Work out the finished part from the listing and answer in its coordinate system (mm). A direction names the side the tool comes from. Coordinates: 2 decimals unless noted, no trailing zeros. Order: outer loops, then holes, each group sorted by start corner. A loop starts at its lowest first (then second) coordinate and runs counter-clockwise, first axis right, second up.
```python
from build123d import *

# Parameters (mm, degrees)
SKETCH1_R           = 1.65
SKETCH1_R_2         = 1.1
SKETCH1_R_3         = 1.4
SKETCH1_R_4         = 11
SKETCH1_W           = 28
SKETCH1_H           = 83
SKETCH1_W_2         = 6.35
SKETCH1_H_2         = 20
SKETCH1_W_3         = 20
SKETCH1_H_3         = 6.35
BOSS_EXTRUDE1_DEPTH = 6.35


with BuildPart() as part:
    # Sketch1 → Boss-Extrude1 (new body)
    with BuildSketch(Plane(origin=(0, 0, 0), x_dir=(1, 0, 0), z_dir=(0, 1, 0))):
        with BuildLine():
            Line((-110, 85), (-2.828427125, 192.171572875))
            ThreePointArc((-2.828427125, 192.171572875), (0, 193.343145751), (2.828427125, 192.171572875))
            Line((2.828427125, 192.171572875), (110, 85))
            Line((110, 85), (110, -85))
            Line((110, -85), (-110, -85))
            Line((-110, -85), (-110, 85))
        make_face()
        with Locations(Location((-39, 10.85, 0), (0, 0, 270))):
            Circle(SKETCH1_R, mode=Mode.SUBTRACT)
        with Locations(Location((-39, -10.85, 0), (0, 0, 90))):
            Circle(SKETCH1_R, mode=Mode.SUBTRACT)
        with Locations(Location((-89.294117647, -69, 0), (0, 0, 270))):
            Circle(SKETCH1_R, mode=Mode.SUBTRACT)
        with Locations(Location((89.294117647, -69, 0), (0, 0, 90))):
            Circle(SKETCH1_R, mode=Mode.SUBTRACT)
        with Locations(Location((-89.294117647, 69, 0), (0, 0, 90))):
            Circle(SKETCH1_R, mode=Mode.SUBTRACT)
        with Locations(Location((89.294117647, 69, 0), (0, 0, 270))):
            Circle(SKETCH1_R, mode=Mode.SUBTRACT)
        with Locations(Location((39, -10.85, 0), (0, 0, 270))):
            Circle(SKETCH1_R, mode=Mode.SUBTRACT)
        with Locations(Location((39, 10.85, 0), (0, 0, 90))):
            Circle(SKETCH1_R, mode=Mode.SUBTRACT)
        with Locations(Location((0, 157, 0), (0, 0, 270))):
            Circle(SKETCH1_R_2, mode=Mode.SUBTRACT)
        with Locations(Location((0, 141.75, 0), (0, 0, 270))):
            Circle(SKETCH1_R_2, mode=Mode.SUBTRACT)
        with Locations(Location((-3, -21, 0), (0, 0, 270))):
            Circle(SKETCH1_R_3, mode=Mode.SUBTRACT)
        with Locations(Location((-3, -70, 0), (0, 0, 270))):
            Circle(SKETCH1_R_3, mode=Mode.SUBTRACT)
        with Locations(Location((58.5, -70, 0), (0, 0, 270))):
            Circle(SKETCH1_R_3, mode=Mode.SUBTRACT)
        with Locations(Location((58.5, -21, 0), (0, 0, 270))):
            Circle(SKETCH1_R_3, mode=Mode.SUBTRACT)
        with Locations(Location((-6.75, 78.125, 0), (0, 0, 270))):
            Circle(SKETCH1_R, mode=Mode.SUBTRACT)
        with Locations(Location((6.75, 78.125, 0), (0, 0, 270))):
            Circle(SKETCH1_R, mode=Mode.SUBTRACT)
        with Locations(Location((6.75, 64.625, 0), (0, 0, 270))):
            Circle(SKETCH1_R, mode=Mode.SUBTRACT)
        with Locations(Location((-6.75, 64.625, 0), (0, 0, 270))):
            Circle(SKETCH1_R, mode=Mode.SUBTRACT)
        with Locations(Location((0, 173, 0), (0, 0, 270))):
            Circle(SKETCH1_R_4, mode=Mode.SUBTRACT)
        with Locations((-83, 0)):
            Rectangle(SKETCH1_W, SKETCH1_H, mode=Mode.SUBTRACT)
        with Locations((-104, 50)):
            Rectangle(SKETCH1_W_2, SKETCH1_H_2, mode=Mode.SUBTRACT)
        with Locations((-104, 0)):
            Rectangle(SKETCH1_W_2, SKETCH1_H_2, mode=Mode.SUBTRACT)
        with Locations((-104, -50)):
            Rectangle(SKETCH1_W_2, SKETCH1_H_2, mode=Mode.SUBTRACT)
        with Locations((50, -77.667136592)):
            Rectangle(SKETCH1_W_3, SKETCH1_H_3, mode=Mode.SUBTRACT)
        with Locations((0, -77.667136592)):
            Rectangle(SKETCH1_W_3, SKETCH1_H_3, mode=Mode.SUBTRACT)
        with Locations((-50, -77.667136592)):
            Rectangle(SKETCH1_W_3, SKETCH1_H_3, mode=Mode.SUBTRACT)
        with Locations((104, -50)):
            Rectangle(SKETCH1_W_2, SKETCH1_H_2, mode=Mode.SUBTRACT)
        with Locations((104, 50)):
            Rectangle(SKETCH1_W_2, SKETCH1_H_2, mode=Mode.SUBTRACT)
        with Locations((104, 0)):
            Rectangle(SKETCH1_W_2, SKETCH1_H_2, mode=Mode.SUBTRACT)
        with Locations((-50, 77.667136592)):
            Rectangle(SKETCH1_W_3, SKETCH1_H_3, mode=Mode.SUBTRACT)
        with Locations((50, 77.667136592)):
            Rectangle(SKETCH1_W_3, SKETCH1_H_3, mode=Mode.SUBTRACT)
        with Locations((83, 0)):
            Rectangle(SKETCH1_W, SKETCH1_H, mode=Mode.SUBTRACT)
    extrude(amount=BOSS_EXTRUDE1_DEPTH)


solid = part.part
```
1. Consider probe 1 along X at (y, z) = (4.75, 21); probe 2 along X at (y, z) = (5.75, -38); probe 3 along X at (y, z) = (6, 58) (3 decimals). Determine where each line is inside the solid, lowest interval first.
2. The mould has two halves that part along Z. Classify faces 3 (the flat face through (110, 3, -1)), 4 (the flat face through (100.825, 3, 0)): released by +Z, released by -Z, zero draft, split by the parting line, or undercut.
3. The part is cut by section C-C (z = -171). Determine the outline of the cut face in (x, y), plus the area to 3 significant figures.
4. For faces 1 (the flat face through (-100.825, 3, 50)), 2 (the flat face through (-110, 3, 1)), determine the directions among +Z, -Z, +X, -X, +Y, -Y from which every point of the face is accessible in a straight line to the end or side of a thin tool.
5. The part is cut by section B-B (z = 35). Determine the outline of the cut face in (x, y), plus the area to 3 significant figures.
6. The part is cut by section D-D (y = 2). Count the separate pieces of the cut face and the enclosed holes in it, plus the area to 3 significant figures.
7. The part is cut by section A-A (x = 81.5). Determine the outline of the cut face in (y, z).
8. Flat-ended cylindrical pins translate along their axes: pin 1 (1 mm diameter, centred on x = -27, y = 1, fed in from -Z); pin 2 (1 mm diameter, centred on y = 3.5, z = -162, fed in from +X). Find the tip coordinate at first contact, or state that the pin passes through.
Worked out:
1. probe 1: x = -110 to -97, -69 to -4.4, -1.6 to 57.1, 59.9 to 69, 97 to 110
1. probe 2: x = -110 to -97, -69 to 69, 97 to 110
1. probe 3: x = -110 to -107.175, -100.825 to 100.825, 107.175 to 110
2. face 3: zero draft
2. face 4: undercut
3. outline: (-24, 0) - (-10.82, 0) - (-10.82, 6.35) - (-24, 6.35) - close; (10.82, 0) - (24, 0) - (24, 6.35) - (10.82, 6.35) - close
3. area: 167 mm2
4. face 1: +Y, -Y
4. face 2: +Z, -Z, -X, +Y, -Y
5. outline: (-110, 0) - (-97, 0) - (-97, 6.35) - (-110, 6.35) - close; (-69, 0) - (69, 0) - (69, 6.35) - (-69, 6.35) - close; (97, 0) - (110, 0) - (110, 6.35) - (97, 6.35) - close
5. area: 1,040 mm2
6. separate pieces: 1
6. enclosed holes: 32
6. area: 42,900 mm2
7. outline: (0, -113.5) - (6.35, -113.5) - (6.35, -41.5) - (0, -41.5) - close; (0, 41.5) - (6.35, 41.5) - (6.35, 85) - (0, 85) - close
8. pin 1: stops at z = -168.5
8. pin 2: stops at x = 33.5
